Geometry check sheet. Reference: the model listing, model coordinates, mm. Face numbers are marked on the shaded views. Coordinates: 2 decimals unless noted, no trailing zeros. Write each loop counter-clockwise with the first axis right and the second up, starting at its lowest first coordinate (ties: lowest second). Pieces come first, ordered by that corner, then holes.
from build123d import *

# Parameters (mm, degrees)
F0_R     = 3.5
F0_R_2   = 1.5
F1_DEPTH = 2
F2_SIZE  = 1.99999
F3_R     = 3
F3_R_2   = 1.5
F4_DEPTH = 4


# Not quite as in the source:
# - a fillet or chamfer is up to 0.001 mm smaller than in the source, because OpenCascade refuses the exact size


with BuildPart() as f1:
    # F0 (on Front) → F1 (new body)
    with BuildSketch(Plane.XZ):
        Circle(F0_R)
        Circle(F0_R_2, mode=Mode.SUBTRACT)
    extrude(amount=F1_DEPTH)

    # F2 (size 2 in the source; OpenCascade refuses exactly that, so slightly less here)
    f2_edges = [f1.edges().sort_by_distance(p)[0] for p in [
        (-1.5, -2, 0),
    ]]
    chamfer(f2_edges, length=F2_SIZE)

    # F3 (on face) → F4 (join)
    with BuildSketch(Plane(origin=(0, 0, 0), x_dir=(-1, 0, 0), z_dir=(0, 1, 0))):
        Circle(F3_R)
        Circle(F3_R_2, mode=Mode.SUBTRACT)
    extrude(amount=F4_DEPTH)


solid = f1.part
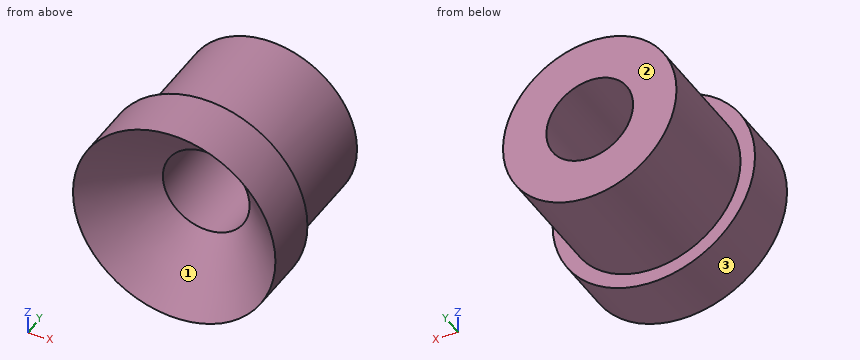
1. Thickness scan on line 1 along Z through (x, y) = (0, 2.55); line 2 along Z through (x, y) = (-1.5, -1.4); line 3 along X through (y, z) = (-1.45, -1.75). Record the ranges inside material, lowest first.
Computed values:
line 1: z = -3 to -1.5, 1.5 to 3
line 2: z = -3.16 to -2.48, 2.48 to 3.16
line 3: x = -3.03 to -2.37, 2.37 to 3.03
2. Sectioned sample at C-C, the plane y = 2.7. Record the boundary of the cut face in (x, z).
Computed values:
outline: circle Ø6 at (0, 0); hole circle Ø3 at (0, 0)
3. Sectioned sample at D-D, the plane y = -1.55. Record the boundary of the cut face in (x, z).
Computed values:
outline: circle Ø7 at (0, 0); hole circle Ø6.1 at (0, 0)
4. Gauge pin test, flat ends, axial feed: pin 1 Ø3 at (x, y) = (0, 2.5) entering from -Z; pin 2 Ø1 at (y, z) = (0, -2) entering from +X; pin 3 Ø2.5 at (x, z) = (0, 0) entering from -Y. Record the tip position at first contact, or that the pin passes through.
Computed values:
pin 1: stops at z = -3
pin 2: stops at x = 3.16
pin 3: passes through
5. Draft check along Y on the marked faces 1, 2 and 3. Enter one of: released by +Y, released by -Y, zero draft, split by the parting line, or undercut.
Computed values:
face 1: released by -Y
face 2: released by +Y
face 3: zero draft
